Can you work these out from the model? Positions are in its coordinate system, mm. A direction names the side the tool comes from. Give positions to 0.01 mm unless a question says otherwise; leave off trailing zeros. Order: outer loops, then holes, each group sorted by start corner. A loop starts at its lowest first (then second) coordinate and runs counter-clockwise, first axis right, second up. Notation, with made-up numbers: M 55,3 L 71,3 A26 ccw 71,23 Z; hole C 31,78 d2. An arc over 180 degrees is marked long. Use one line per item in the form item = value. Start each with the question number.
1. For faces 1 (the face through (474.435, -105.353, 0.991)), 2 (the face through (20, 277, 45)), which set-ups out of +Z, -Z, +X, -X, +Y, -Y let a thin tool reach every point of the face, with its end or its side?
2. Will these pins go through, and if not, where does the flat tip stop? P1, Ø10, axis at x = 381.5, y = -181, coming from the -Z side; P2, Ø6, axis at x = -290, z = 26.5, coming from the +Y side; P3, Ø3, axis at y = 250, z = 67, coming from the +X side; P4, Ø9, axis at y = 249, z = 38, coming from the +X side.
3. We'd pull the mould along X, two halves only. Please class faces 3 (the face through (-7, 7, 0)), 4 (the face through (-139.67, 443.53, 49.72)), 5 (the face through (-150.61, 478.27, 17.99)): +X half, -X half, draft (parallel to the pull), parting line (faces both ways), or undercut.
4. I want a section at B-B, the plane y = 0. List the corners of the cut face in (x, z) for me.
5. I want a section at A-A, the plane x = 0. List the corners of the cut face in (y, z) for me.
6. I need wall thicknesses on L1, parallel to X at y = 0, z = 53; L2, parallel to X at y = 120, z = 45. Which ranges of each line are inside material? Lowest first, please.
```python
from build123d import *

# Parameters (mm, degrees)
BOSS_EXTRUDE1_DEPTH = 30
FILLET1_R           = 60
FILLET2_R           = 10


with BuildPart() as part:
    # Sketch1 → Revolve1 (revolve)
    with BuildSketch(Plane(origin=(0, 0, 0), x_dir=(0, 0, -1), z_dir=(1, 0, 0))):
        Polygon((0, 0), (0, 485), (-15.849364905, 500.849364905), (-50, 510), (-70, 510), (-70, 465), (-30, 465), (-30, 100), (-90, 100), (-90, 0), (-30, 0), align=None)
    revolve(axis=Axis((0, 0, 0), (0, 0, 1)))

    # Sketch2 → Boss-Extrude1 (add)
    with BuildSketch(Plane.XY.offset(30)):
        with BuildLine():
            Line((-20, 464.569693372), (-20, 97.979589711))
            ThreePointArc((-20, 97.979589711), (0, 100), (20, 97.979589711))
            Line((20, 97.979589711), (20, 464.569693372))
            ThreePointArc((20, 464.569693372), (0, 465), (-20, 464.569693372))
        make_face()
    extrude(amount=BOSS_EXTRUDE1_DEPTH)

    # Fillet1
    fillet1_edges = [part.edges().sort_by_distance(p)[0] for p in [
        (-20, 464.569693372, 45),
    ]]
    fillet(fillet1_edges, radius=FILLET1_R)

    # Fillet2
    fillet2_edges = [part.edges().sort_by_distance(p)[0] for p in [
        (20, 464.569693372, 45),
        (-20, 97.979589711, 45),
        (20, 97.979589711, 45),
    ]]
    fillet(fillet2_edges, radius=FILLET2_R)


solid = part.part
```
Check result:
q1.face_1 = -Z
q1.face_2 = +Z
q2.P1 = 0
q2.P2 = 414.16
q2.P3 = 445.36
q2.P4 = 444.26
q3.face_3 = draft
q3.face_4 = undercut
q3.face_5 = parting line
q4.outline = M -510,50 L -500.85,15.85 L -485,0 L 485,0 L 500.85,15.85 L 510,50 L 510,70 L 465,70 L 465,30 L 100,30 L 100,90 L -100,90 L -100,30 L -465,30 L -465,70 L -510,70 Z
q5.outline = M -510,50 L -500.85,15.85 L -485,0 L 485,0 L 500.85,15.85 L 510,50 L 510,70 L 465,70 L 465,60 L 100,60 L 100,90 L -100,90 L -100,30 L -465,30 L -465,70 L -510,70 Z
q6.L1 = -510 to -465, -100 to 100, 465 to 510
q6.L2 = -494.3 to -449.25, -20 to 20, 449.25 to 494.3
